from build123d import *

# Parameters (mm, degrees)
F0_R      = 40
F0_R_2    = 35
F1_DEPTH  = 50
F2_R      = 45
F2_R_2    = 35
F3_DEPTH  = 15
F4_R      = 5
F6_R      = 40
F6_R_2    = 37.5
F7_DEPTH  = 10
F9_DEPTH  = 5
F11_DEPTH = 5


with BuildPart() as f1:
    # F0 (on Front) → F1 (new body)
    with BuildSketch(Plane.XZ):
        Circle(F0_R)
        Circle(F0_R_2, mode=Mode.SUBTRACT)
    extrude(amount=F1_DEPTH)

    # F2 (on Front) → F3 (join)
    with BuildSketch(Plane.XZ):
        Circle(F2_R)
        Circle(F2_R_2, mode=Mode.SUBTRACT)
    extrude(amount=F3_DEPTH)

    # F4
    f4_edges = [f1.edges().sort_by_distance(p)[0] for p in [
        (-35, 0, 0),
    ]]
    fillet(f4_edges, radius=F4_R)

    # F6 (on offset) → F7 (cut)
    with BuildSketch(Plane.XZ.offset(45)):
        Circle(F6_R)
        Circle(F6_R_2, mode=Mode.SUBTRACT)
    extrude(amount=-F7_DEPTH, mode=Mode.SUBTRACT)

    # F8 (on offset) → F9 (join)
    with BuildSketch(Plane.XZ.offset(45)):
        with BuildLine():
            Line((23.4356336296, 9.2309236786), (33.7607767689, 9.2309236786))
            ThreePointArc((33.7607767689, 9.2309236786), (1.5790357434, 34.9643625156), (-32.7912801838, 12.2365004764))
            Line((-32.7912801838, 12.2365004764), (-21.8026206791, 12.2365004764))
            ThreePointArc((-21.8026206791, 12.2365004764), (1.7678734782, 25.0531540072), (23.4356336296, 9.2309236786))
        make_face()
    extrude(amount=-F9_DEPTH)

    # F10 (on offset) → F11 (join)
    with BuildSketch(Plane.XZ.offset(45)):
        with BuildLine():
            Line((-24.3510891636, -7.7079934607), (-34.1406918033, -7.7079934607))
            ThreePointArc((-34.1406918033, -7.7079934607), (0, -35), (34.1406918033, -7.7079934607))
            Line((34.1406918033, -7.7079934607), (24.5616502176, -7.7079934607))
            ThreePointArc((24.5616502176, -7.7079934607), (0.105280527, -25.6222077044), (-24.3510891636, -7.7079934607))
        make_face()
    extrude(amount=-F11_DEPTH)


solid = f1.part
Here's how the part is built. I have some questions about the finished solid (model axes, mm). A direction names the side the tool comes from. Coordinates: 2 decimals unless noted, no trailing zeros. Order: outer loops, then holes, each group sorted by start corner. A loop starts at its lowest first (then second) coordinate and runs counter-clockwise, first axis right, second up.
Item 1: If we section it at A-A on z = 0: List the corners of the cut face in (x, y) for me.
Result sheet:
outline: (-45, -15) - (-40, -15) - (-40, -35) - (-37.5, -35) - (-37.5, -45) - (-40, -45) - (-40, -50) - (-35, -50) - (-35, -5) arc R5 ccw to (-40, 0) - (-45, 0) - close; (35, -50) - (40, -50) - (40, -45) - (37.5, -45) - (37.5, -35) - (40, -35) - (40, -15) - (45, -15) - (45, 0) - (40, 0) arc R5 ccw to (35, -5) - close
Item 2: If we mould it in two halves opening along X, with no side actions, what happens to faces 1 (the face through (29, -43, 9.231)), 2 (the face through (-8.67, -47.46, -39.05)), 3 (the face through (-30.2, 0, -26.5))? For each: +X half, -X half, draft (parallel to the pull), parting line (faces both ways), or undercut.
Result sheet:
face 1: undercut
face 2: parting line
face 3: draft
Item 3: For faces 4 (the face through (-8.67, -24.86, -39.05)), 5 (the face through (12, -45, 36)), 6 (the face through (0, -40, 28)), 7 (the face through (-29, -43, -7.708)), which set-ups out of +Z, -Z, +X, -X, +Y, -Y let a thin tool reach every point of the face, with its end or its side?
Result sheet:
face 4: -Y
face 5: none
face 6: +Y
face 7: +Y, -Y
Item 4: For P1, Ø5.5, axis at x = -29.5, y = -43, coming from the +Z side; P2, Ø5.5, axis at x = 27, y = -41.5, coming from the -Z side; P3, Ø12, axis at y = -26.5, z = 33, coming from the -X side, each with a flat end and sliding along its axis, tell me the tip position at first contact or that it passes through.
Result sheet:
P1: stops at z = 28.94
P2: stops at z = -28.6
P3: stops at x = -29.51
Item 5: If we section it at C-C on y = -16.5: List the corners of the cut face in (x, z) for me, plus the area to 3 significant figures.
Result sheet:
outline: circle Ø80 at (0, 0); hole circle Ø70 at (0, 0)
area: 1,180 mm2
Item 6: I need wall thicknesses on line 1 (Z direction, x = 0, y = -31); line 2 (Z direction, x = 0, y = -38.5); line 3 (Y direction, x = 7.5, z = -31.5). Which ranges of each line are inside material? Lowest first, please.
Result sheet:
line 1: z = -40 to -35, 35 to 40
line 2: z = -37.5 to -35, 35 to 37.5
line 3: y = -45 to -40
